```python
from build123d import *

# Parameters (mm, degrees)
SKETCH1_W           = 27.2
SKETCH1_H           = 23.9
BOSS_EXTRUDE1_DEPTH = 30
SHELL1_T            = -3.5
BOSS_EXTRUDE2_DEPTH = 13.7
SHELL3_START        = -10.194612797
SHELL3_DEPTH        = 20.389225594
FILLET2_R           = 2
SKETCH3_R           = 2.1
CUT_EXTRUDE1_DEPTH  = 100.698379758
FILLET3_R           = 10
SKETCH4_W           = 27.4
SKETCH4_H           = 4.712888426
CUT_EXTRUDE2_DEPTH  = 89.262138497


# Read off the part's stored shape, not the designer's step: Shell3
with BuildPart() as part:
    # Sketch1 → Boss-Extrude1 (new, symmetric)
    with BuildSketch(Plane(origin=(0, 0, 0), x_dir=(0, 0, -1), z_dir=(1, 0, 0))):
        Rectangle(SKETCH1_W, SKETCH1_H)
    extrude(amount=BOSS_EXTRUDE1_DEPTH, both=True)

    # Shell1
    shell1_openings = [part.faces().sort_by_distance(p)[0] for p in [
        (30, 0, 0),
        (-30, 0, 0),
        (0, 11.95, 0),
    ]]
    offset(amount=SHELL1_T, openings=shell1_openings, kind=Kind.INTERSECTION)

    # Sketch2 → Boss-Extrude2 (add, symmetric)
    with BuildSketch(Plane(origin=(0, 0, 0), x_dir=(0, 0, -1), z_dir=(1, 0, 0))):
        Polygon((4.94675733, -11.95), (42.229225693, -65.194882879), (61.479298734, -51.715836625), (13.6, 16.662888426), (10.1, 16.662888426), (10.1, 11.95), (13.6, 11.95), (13.6, -11.95), align=None)
    extrude(amount=BOSS_EXTRUDE2_DEPTH, both=True)

    # Shell3 outline → Shell3 (cut)
    with BuildSketch(Plane.YZ.offset(SHELL3_START)):
        Polygon((13.157501223, -16.054498544), (13.157501223, -13.605387203), (-11.955387203, -13.605387203), (-11.955387203, -9.229817112), (-63.184275379, -45.100670786), (-51.715836625, -61.479298734), align=None)
    extrude(amount=SHELL3_DEPTH, mode=Mode.SUBTRACT)

    # Fillet2
    fillet2_edges = [part.edges().sort_by_distance(p)[0] for p in [
        (0, -11.95, 13.6),
    ]]
    fillet(fillet2_edges, radius=FILLET2_R)

    # Sketch3 → Cut-Extrude1 (cut, through all)
    with BuildSketch(Plane(origin=(13.7, 0, 0), x_dir=(0, 0, -1), z_dir=(1, 0, 0))):
        with Locations((49.272743236, -51.717536678)):
            Circle(SKETCH3_R)
        with Locations((37.801214509, -35.334495792)):
            Circle(SKETCH3_R)
        with Locations((26.329685782, -18.951454906)):
            Circle(SKETCH3_R)
    extrude(amount=-CUT_EXTRUDE1_DEPTH, mode=Mode.SUBTRACT)

    # Fillet3
    fillet3_edges = [part.edges().sort_by_distance(p)[0] for p in [
        (0, -11.95, -4.94675733),
    ]]
    fillet(fillet3_edges, radius=FILLET3_R)

    # Sketch4 → Cut-Extrude2 (cut, through all)
    with BuildSketch(Plane.XY.offset(-10.1)):
        with Locations((0, 14.306444213)):
            Rectangle(SKETCH4_W, SKETCH4_H)
    extrude(amount=-CUT_EXTRUDE2_DEPTH, mode=Mode.SUBTRACT)


solid = part.part
```
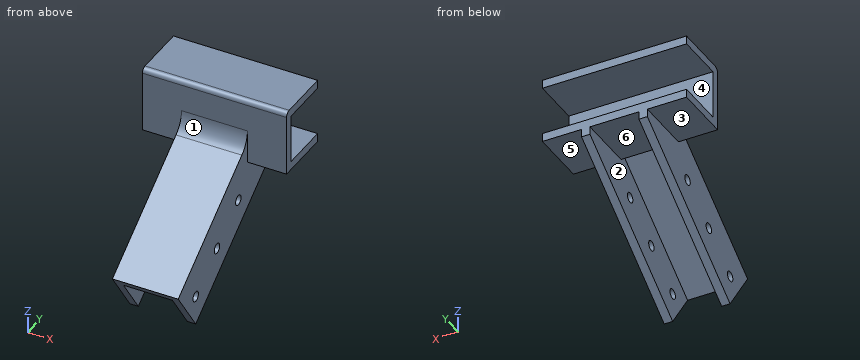
Geometry: final body of the model. Coordinates: model frame, mm. Face numbers are marked on the shaded views. A direction names the side the tool comes from. Round coordinates to 2 decimals unless told otherwise and drop trailing zeros. Loops run counter-clockwise (first coordinate to the right, second up) from the corner with the lowest first, then second, coordinate; pieces in that order, holes last. Notation, with made-up numbers: (-11, 89) -> (2, 89) arc R6 cw to (2, 100) -> close; hole circle Ø4 at (35.25, 13.5). An arc over 180 degrees is marked (long way). Use one line per item in the form item = value. Start each with the question number.
1) Access query for the marked faces 3, 4, 5 and 6. Directions: +Z, -Z, +X, -X, +Y, -Y. A direction counts if a zero-diameter tool reaches every point of the face in a straight line with its end or side. Return the directions, or none.
2) Draft query along X for the marked faces 1 and 2. Return one class per face: released by +X, released by -X, zero draft, split by the parting line, or undercut.
3) Line query: L1, parallel to X at y = -32.5, z = -33; L2, parallel to Z at x = -14, y = 0; L3, parallel to Y at x = 21.5, z = -1.5. Output: solid intervals per line, ascending.
4) Section C-C on y = -13.5. Output: boundary loops of the cut face in (x, z), then the cut area to 3 significant figures.
5) Section D-D on z = -34.5. Output: boundary loops of the cut face in (x, y), then the cut area to 3 significant figures.
6) Section B-B on x = 3. Output: boundary loops of the cut face in (y, z).
7) Section A-A on y = 1.5. Output: boundary loops of the cut face in (x, z), then the cut area to 3 significant figures.
8) First-contact query: P1, Ø13, axis at x = -24, y = 3, coming from the -Z side; P2, Ø3.5, axis at x = 0, z = -11, coming from the -Y side; P3, Ø3, axis at y = -47.5, z = -38.5, coming from the -X side. Flat tips, straight axial feed; report the tip coordinate or a pass-through.
Response:
q1.face_3 = -Z, -X, +Y, -Y
q1.face_4 = +X, -X, +Y
q1.face_5 = -Z, +X, +Y, -Y
q1.face_6 = -Z, +Y
q2.face_1 = zero draft
q2.face_2 = undercut
q3.L1 = -13.7 to -10.19, 10.19 to 13.7
q3.L2 = -13.6 to -10.1, 10.1 to 13.6
q3.L3 = -11.95 to -8.45
q4.outline = (-13.7, -34.72) -> (-10.19, -34.72) -> (-10.19, -10.31) -> (10.19, -10.31) -> (10.19, -34.72) -> (13.7, -34.72) -> (13.7, -5.09) -> (-13.7, -5.09) -> close
q4.area = 314 mm^2
q5.outline = (-13.7, -54.16) -> (13.7, -54.16) -> (13.7, -13.19) -> (10.19, -13.19) -> (10.19, -48.04) -> (-10.19, -48.04) -> (-10.19, -13.19) -> (-13.7, -13.19) -> close
q5.area = 412 mm^2
q6.outline = (-65.19, -42.23) -> (-63.18, -45.1) -> (-11.96, -9.23) -> (-11.96, -13.61) -> (11.95, -13.61) -> (11.95, -10.1) -> (-8.45, -10.1) -> (-8.45, 10.1) -> (11.95, 10.1) -> (11.95, 13.6) -> (-9.95, 13.6) arc R2 ccw to (-11.95, 11.6) -> (-11.95, 0.26) arc R10 cw to (-16.21, -7.93) -> close
q7.outline = (-30, -13.6) -> (-13.7, -13.6) -> (-13.7, -24.22) -> (-10.19, -24.22) -> (-10.19, -13.61) -> (10.19, -13.61) -> (10.19, -24.22) -> (13.7, -24.22) -> (13.7, -13.6) -> (30, -13.6) -> (30, -10.1) -> (-30, -10.1) -> close; (-30, 10.1) -> (30, 10.1) -> (30, 13.6) -> (-30, 13.6) -> close
q7.area = 495 mm^2
q8.P1 = -13.6
q8.P2 = -23.09
q8.P3 = -13.7
